```python
from build123d import *

# Parameters (mm, degrees)
BOSS_EXTRUDE1_DEPTH     = 38.1
CUT_EXTRUDE1_DEPTH      = 31.75
CUT_EXTRUDE1_DEPTH_BACK = 31.75
FILLET1_R               = 6.35
SKETCH3_R               = 2.286
CUT_EXTRUDE2_DEPTH      = 83.366623246


with BuildPart() as part:
    # Sketch1 → Boss-Extrude1 (new, symmetric)
    with BuildSketch(Plane(origin=(0, 0, 0), x_dir=(1, 0, 0), z_dir=(0, 1, 0))):
        with BuildLine():
            Line((-12.7, -3.175), (-12.7, -28.575))
            Line((-12.7, -28.575), (-9.525, -28.575))
            Line((-9.525, -28.575), (-9.525, -22.225))
            Line((-9.525, -22.225), (3.922177061, -2.70146874))
            ThreePointArc((3.922177061, -2.70146874), (2.990880149, 3.706216694), (-3.468948889, 3.263096667))
            Line((-3.468948889, 3.263096667), (-9.525, -3.175))
            Line((-9.525, -3.175), (-12.7, -3.175))
        make_face()
    extrude(amount=BOSS_EXTRUDE1_DEPTH, both=True)

    # Sketch2 → Cut-Extrude1 (cut, two sides: drawn at the far end of the back side and taken through both)
    with BuildSketch(Plane(origin=(0, 0, 0), x_dir=(1, 0, 0), z_dir=(0, 1, 0)).offset(-CUT_EXTRUDE1_DEPTH_BACK)):
        with BuildLine():
            Line((-3.468948889, 3.263096667), (-9.525, -3.175))
            Line((-9.525, -3.175), (-9.525, -22.225))
            Line((-9.525, -22.225), (3.922177061, -2.70146874))
            ThreePointArc((3.922177061, -2.70146874), (2.990880149, 3.706216694), (-3.468948889, 3.263096667))
        make_face()
    extrude(amount=CUT_EXTRUDE1_DEPTH + CUT_EXTRUDE1_DEPTH_BACK, mode=Mode.SUBTRACT)

    # Fillet1
    fillet1_edges = [part.edges().sort_by_distance(p)[0] for p in [
        (-11.1125, -38.1, 28.575),
        (-11.1125, 38.1, 28.575),
    ]]
    fillet(fillet1_edges, radius=FILLET1_R)

    # Sketch3 → Cut-Extrude2 (cut, through all)
    with BuildSketch(Plane(origin=(0, 38.1, 0), x_dir=(1, 0, 0), z_dir=(0, 1, 0))):
        with Locations(Location((0, 0, 0), (0, 0, 270))):
            Circle(SKETCH3_R)
    extrude(amount=-CUT_EXTRUDE2_DEPTH, mode=Mode.SUBTRACT)


solid = part.part
```
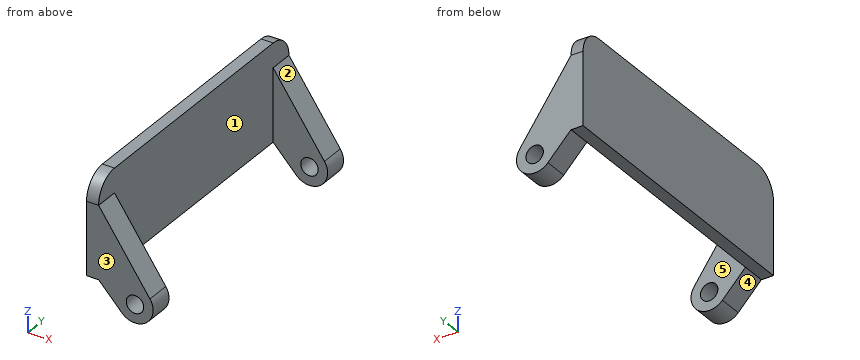
CAD build for the part. Positions are in the model's coordinates, mm. Face numbers are marked on the shaded views. A direction names the side the tool comes from. Coordinates: 2 decimals unless noted, no trailing zeros. Loops run counter-clockwise (first coordinate to the right, second up) from the corner with the lowest first, then second, coordinate; pieces in that order, holes last. Notation, with made-up numbers: (77.25, 72.5) - (82.25, 72.5) arc R33 cw to (82.25, 106.5) - close; hole circle Ø8 at (23.25, -31.75). An arc over 180 degrees is marked (long way). Return JSON: item names as keys, results as strings.
1. Band-saw the part on D-D (z = 6). Give the cut face in (x, y) (3 decimals), and give its area (3 significant figures).
Result:
{"outline": "(-12.7, -38.1) - (1.65, -38.1) - (1.65, -31.75) - (-9.525, -31.75) - (-9.525, 31.75) - (1.65, 31.75) - (1.65, 38.1) - (-12.7, 38.1) - close", "area": "384 mm2"}
2. Drop flat-ended pins along their axis: pin 1 (12.5 mm diameter, centred on y = -12.5, z = 10, fed in from +X) (3 decimals); pin 2 (3.5 mm diameter, centred on x = -11, y = 5, fed in from -Z) (3 decimals). Give the stop position or say it passes through.
Result:
{"pin 1": "stops at x = -9.525", "pin 2": "stops at z = 3.175"}
3. 3-axis set-ups, long thin cutter, end or side, ignore diameter. For the marked faces 4 and 5: which of +Z, -Z, +X, -X, +Y, -Y reach the whole face in a straight line?
Result:
{"face 4": "-Z, -X, +Y, -Y", "face 5": "+Z, -Z, +X"}
4. Probe L1, parallel to Y at x = 3, z = 2; L2, parallel to X at y = 16, z = 12.5 (3 decimals). List the from-to ranges inside material, lowest first. Write a range as from..to.
Result:
{"L1": "y = -38.1..-31.75, 31.75..38.1", "L2": "x = -12.7..-9.525"}
5. Band-saw the part on B-B (x = 0). Give the cut face in (y, z), and give its area (3 significant figures).
Result:
{"outline": "(-38.1, -4.76) - (-31.75, -4.76) - (-31.75, -2.29) - (-38.1, -2.29) - close; (-38.1, 2.29) - (-31.75, 2.29) - (-31.75, 8.4) - (-38.1, 8.4) - close; (31.75, -4.76) - (38.1, -4.76) - (38.1, -2.29) - (31.75, -2.29) - close; (31.75, 2.29) - (38.1, 2.29) - (38.1, 8.4) - (31.75, 8.4) - close", "area": "109 mm2"}
6. Mould opens along Y. For the marked faces 1, 2 and 3 say: released by +Y, released by -Y, zero draft, split by the parting line, or undercut.
Result:
{"face 1": "undercut", "face 2": "zero draft", "face 3": "released by -Y"}
7. Band-saw the part on A-A (x = -4.75). Give the cut face in (y, z), and give its area (3 significant figures).
Result:
{"outline": "(-38.1, -1.9) - (-31.75, -1.9) - (-31.75, 15.29) - (-38.1, 15.29) - close; (31.75, -1.9) - (38.1, -1.9) - (38.1, 15.29) - (31.75, 15.29) - close", "area": "218 mm2"}
8. Band-saw the part on C-C (z = 0). Give the cut face in (x, y).
Result:
{"outline": "(-6.54, -38.1) - (-2.29, -38.1) - (-2.29, -31.75) - (-6.54, -31.75) - close; (-6.54, 31.75) - (-2.29, 31.75) - (-2.29, 38.1) - (-6.54, 38.1) - close; (2.29, -38.1) - (4.76, -38.1) - (4.76, -31.75) - (2.29, -31.75) - close; (2.29, 31.75) - (4.76, 31.75) - (4.76, 38.1) - (2.29, 38.1) - close"}
